Input: dimensioned drawing with shaded views. Units: mm. Origin: part minimum x, y, z. A direction names the side the tool comes from. Give positions to 0.01 mm unless a question says otherwise; leave off trailing zeros. Write each loop counter-clockwise with the first axis right and the second up, starting at its lowest first coordinate (ties: lowest second). Pieces come first, ordered by that corner, then holes. Notation, with made-up numbers: (18.5, 5) -> (44.5, 5) arc R31 ccw to (44.5, 29) -> close; hole circle Ø5 at (77.25, 44.25). An arc over 180 degrees is marked (long way). Return JSON: item names as keys, results as strings. Group by question number.
Item 1: Line query: line 1 (Y direction, x = 8, z = 1.4); line 2 (X direction, y = 5.5, z = 26.5); line 3 (Z direction, x = 1.5, y = 8). Output: solid intervals per line, ascending. Write a range as [from, to].
Item 2: Pin query (flat end, axial travel): P1, Ø14, axis at y = 11, z = 21.5, coming from the -X side. Return the tip coordinate at first contact, or that it passes through.
Item 3: Section A-A, the plane y = 7. Return loops of the section in (x, z), then the cut area to 3 significant figures.
Item 4: Section C-C, the plane x = 18.75. Return loops of the section in (y, z), then the cut area to 3 significant figures.
Item 5: Set-up query: the marked faces 1 and 2. Return all of +Z, -Z, +X, -X, +Y, -Y with unobstructed straight access to the full face (end or side cutting, diameter ignored); none if empty.
Item 6: Section B-B, the plane x = 8. Return loops of the section in (y, z).
Item 7: Section D-D, the plane z = 27.5. Return loops of the section in (x, y).
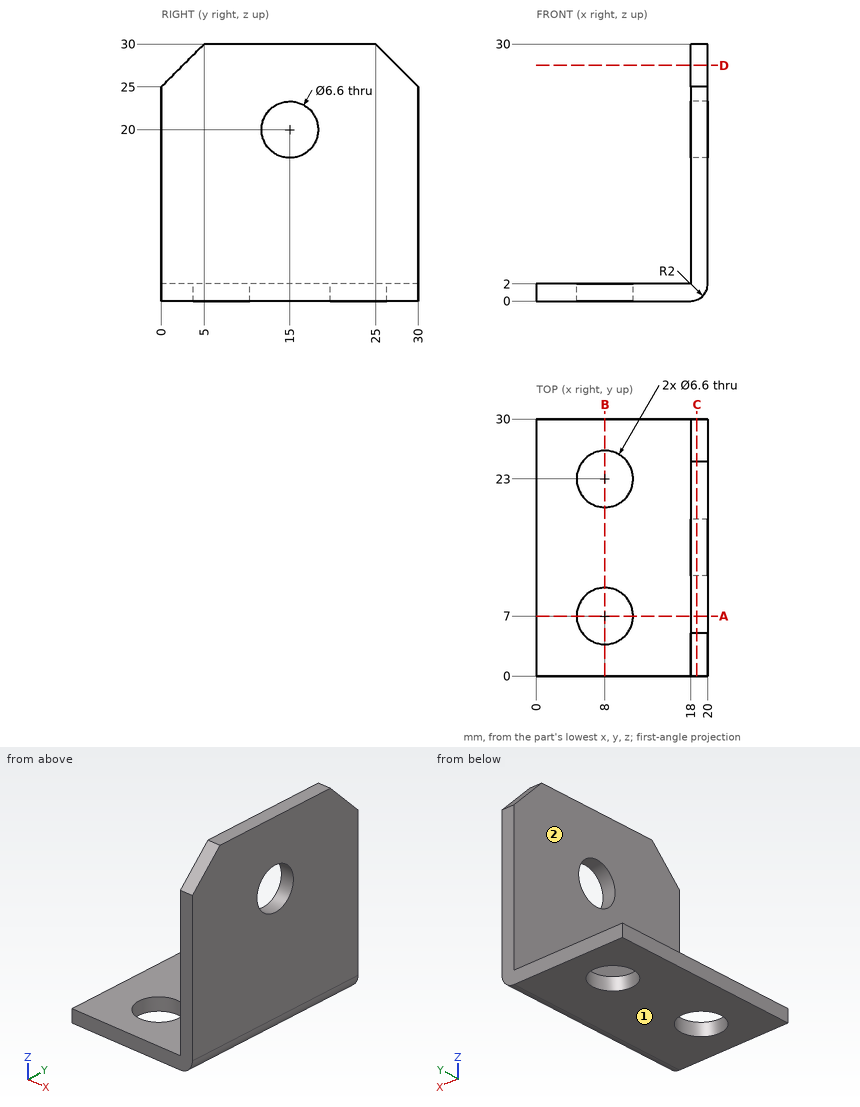
Answer below:
{
 "1": {"line 1": "y = [0, 3.7], [10.3, 19.7], [26.3, 30]", "line 2": "x = [18, 20]", "line 3": "z = [0, 2]"},
 "2": {"P1": "stops at x = 18"},
 "3": {"outline": "(0, 0) -> (4.7, 0) -> (4.7, 2) -> (0, 2) -> close; (11.3, 0) -> (18, 0) arc R2 ccw to (20, 2) -> (20, 30) -> (18, 30) -> (18, 2) -> (11.3, 2) -> close", "area": "81.9 mm2"},
 "4": {"outline": "(0, 0.15) -> (30, 0.15) -> (30, 25) -> (25, 30) -> (5, 30) -> (0, 25) -> close; hole circle Ø6.6 at (15, 20)", "area": "836 mm2"},
 "5": {"face 1": "-Z, +X, -X, +Y, -Y", "face 2": "+Z, -X, +Y, -Y"},
 "6": {"outline": "(0, 0) -> (3.7, 0) -> (3.7, 2) -> (0, 2) -> close; (10.3, 0) -> (19.7, 0) -> (19.7, 2) -> (10.3, 2) -> close; (26.3, 0) -> (30, 0) -> (30, 2) -> (26.3, 2) -> close"},
 "7": {"outline": "(18, 2.5) -> (20, 2.5) -> (20, 27.5) -> (18, 27.5) -> close"}
}
